Can you work these out from the model? Positions are in its coordinate system, mm. Face numbers are marked on the shaded views. A direction names the side the tool comes from. Give positions to 0.01 mm unless a question says otherwise; leave off trailing zeros. Order: outer loops, then holes, each group sorted by start corner. A loop starts at its lowest first (then second) coordinate and runs counter-clockwise, first axis right, second up. Notation, with made-up numbers: M 86,-29.75 L 132,-29.75 A32 cw 132,0.25 Z; hole C 81,64 d7. An arc over 180 degrees is marked long. Use one line per item in the form item = value. Start each with the question number.
1. We'd pull the mould along X, two halves only. Please class the marked faces 3, 4, 5 and 6: +X half, -X half, draft (parallel to the pull), parting line (faces both ways), or undercut.
2. I want a section at A-A, the plane x = -22. List the corners of the cut face in (y, z) for me, and give its area (3 significant figures).
3. Will this pin go through, and if not, where does the flat tip stop? P1, Ø1.5, axis at x = -2.5, z = 1, coming from the -Y side.
4. I want a section at B-B, the plane x = 32.5. List the corners of the cut face in (y, z) for me, and give its area (3 significant figures).
5. For the marked faces 1 and 2, which set-ups out of +Z, -Z, +X, -X, +Y, -Y let a thin tool reach every point of the face, with its end or its side?
6. I need wall thicknesses on L1, parallel to X at y = -0.2, z = 0.65; L2, parallel to X at y = -1.9, z = 1.35; L3, parallel to X at y = -2.2, z = -0.2. Which ranges of each line are inside material? Lowest first, please.
```python
from build123d import *

# Parameters (mm, degrees)
BOSS_EXTRUDE1_DEPTH       = 36.4
FILLET3_R                 = 2.5
CUT_EXTRUDE5_DEPTH        = 72.8
BOSS_EXTRUDE2_DEPTH       = 72.8
M2X0_4_TAPPED_HOLE1_D     = 1.6
M2X0_4_TAPPED_HOLE1_DEPTH = 3.6
M2X0_4_TAPPED_HOLE1_TIP   = 0.480688495
FILLET4_R                 = 2.5
SKETCH4_W                 = 15
SKETCH4_H                 = 4.7
CUT_EXTRUDE4_DEPTH        = 5
BOSS_EXTRUDE6_DEPTH       = 3
BOSS_EXTRUDE7_DEPTH       = 3


with BuildPart() as part:
    # Sketch1 → Boss-Extrude1 (new body, symmetric)
    with BuildSketch(Plane(origin=(0, 0, 0), x_dir=(0, 0, -1), z_dir=(1, 0, 0))):
        Polygon((0, -3.2), (-2, -1.2), (-2, 3.2), (0, 3.2), align=None)
    extrude(amount=BOSS_EXTRUDE1_DEPTH, both=True)

    # Fillet3
    fillet3_edges = [part.edges().sort_by_distance(p)[0] for p in [
        (-36.4, 3.2, 1),
        (36.4, 3.2, 1),
    ]]
    fillet(fillet3_edges, radius=FILLET3_R)

    # Sketch5 → Cut-Extrude5 (cut)
    with BuildSketch(Plane.ZY.offset(36.4)):
        Polygon((0, -2.7), (2, -0.7), (2, -1.2), (0, -3.2), align=None)
    extrude(amount=-CUT_EXTRUDE5_DEPTH, mode=Mode.SUBTRACT)

    # Sketch7 → Boss-Extrude2 (add)
    with BuildSketch(Plane.ZY.offset(36.4)):
        Polygon((0, -2.7), (-1, -1.7), (-1, 3.2), (0, 3.2), align=None)
    extrude(amount=-BOSS_EXTRUDE2_DEPTH)

    # M2x0.4 Tapped Hole1
    with Locations(Plane.XY.offset(2)):
        with Locations((-22, -0.2), (22, -0.2), (0, -0.2)):
            Hole(M2X0_4_TAPPED_HOLE1_D / 2, depth=M2X0_4_TAPPED_HOLE1_DEPTH)
            with Locations((0, 0, -(M2X0_4_TAPPED_HOLE1_DEPTH + M2X0_4_TAPPED_HOLE1_TIP / 2))):  # 118° drill point
                Cone(0, M2X0_4_TAPPED_HOLE1_D / 2, M2X0_4_TAPPED_HOLE1_TIP, mode=Mode.SUBTRACT)

    # Fillet4
    fillet4_edges = [part.edges().sort_by_distance(p)[0] for p in [
        (36.4, 3.2, -0.5),
        (-36.4, 3.2, -0.5),
    ]]
    fillet(fillet4_edges, radius=FILLET4_R)

    # Sketch4 → Cut-Extrude4 (cut, symmetric)
    with BuildSketch(Plane.XY):
        with Locations((0, -0.85)):
            Rectangle(SKETCH4_W, SKETCH4_H)
    extrude(amount=CUT_EXTRUDE4_DEPTH, both=True, mode=Mode.SUBTRACT)

    # Sketch11 → Boss-Extrude6 (add)
    with BuildSketch(Plane(origin=(36.4, 0, 0), x_dir=(0, 0, -1), z_dir=(1, 0, 0))):
        Polygon((0, -2.7), (-1, -2.7), (-2, -1.7), (-2, -0.7), align=None)
    extrude(amount=-BOSS_EXTRUDE6_DEPTH)

    # Sketch12 → Boss-Extrude7 (add)
    with BuildSketch(Plane.ZY.offset(-7.5)):
        Polygon((0, -2.7), (1, -2.7), (2, -1.7), (2, -0.7), align=None)
    extrude(amount=-BOSS_EXTRUDE7_DEPTH)

    # Mirror7: part across plane


with BuildPart() as part_1:
    add(part.part)
    add(part.part.mirror(Plane(origin=(0, 0, 0), x_dir=(0, 0, 1), z_dir=(1, 0, 0))))


solid = part_1.part
```
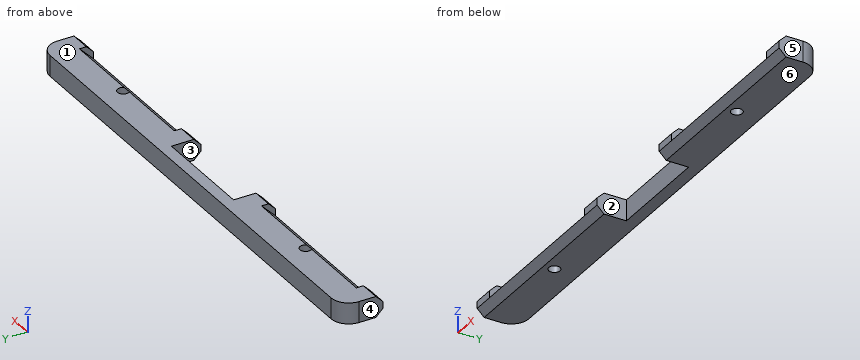
Check result:
q1.face_3 = undercut
q1.face_4 = -X half
q1.face_5 = +X half
q1.face_6 = draft
q2.outline = M -2.7,0 L -1.7,-1 L -1,-1 L -1,1.7 Z; M 0.6,-1 L 3.2,-1 L 3.2,2 L 0.6,2 Z
q2.area = 10.4 mm2
q3.P1 = 1.5
q4.outline = M -2.7,0 L -1.7,-1 L 3.2,-1 L 3.2,2 L -0.7,2 Z
q4.area = 15.2 mm2
q5.face_1 = +Z, +X, -X, +Y, -Y
q5.face_2 = +Z, -Z, -Y
q6.L1 = -36.4 to -22.8, -21.2 to -7.5, 7.5 to 21.2, 22.8 to 36.4
q6.L2 = -36.4 to -33.4, -10.5 to -7.5, 7.5 to 10.5, 33.4 to 36.4
q6.L3 = -36.4 to -7.5, 7.5 to 36.4
